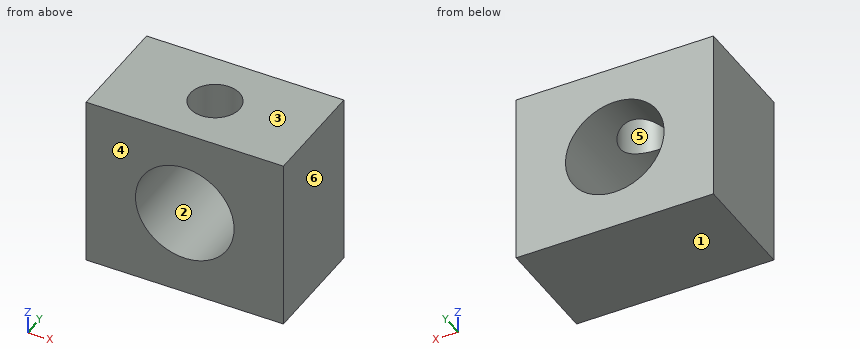
```python
from build123d import *

# Parameters (mm, degrees)
F0_W     = 80
F0_H     = 70
F1_DEPTH = 45
F2_R     = 20
F3_DEPTH = 45.001
F4_R     = 10
F5_DEPTH = 25


with BuildPart() as f1:
    # F0 (on Front) → F1 (new body)
    with BuildSketch(Plane.XZ):
        Rectangle(F0_W, F0_H)
    extrude(amount=-F1_DEPTH)

    # F2 (on face) → F3 (cut, through all)
    with BuildSketch(Plane.XZ):
        Circle(F2_R)
    extrude(amount=-F3_DEPTH, mode=Mode.SUBTRACT)

    # F4 (on face) → F5 (cut)
    with BuildSketch(Plane.XY.offset(35)):
        with Locations((0, 22.5)):
            Circle(F4_R)
    extrude(amount=-F5_DEPTH, mode=Mode.SUBTRACT)


solid = f1.part
```
Geometry: final body of the model. Coordinates: model frame, mm. Face numbers are marked on the shaded views. A direction names the side the tool comes from. Coordinates: 2 decimals unless noted, no trailing zeros. Write each loop counter-clockwise with the first axis right and the second up, starting at its lowest first coordinate (ties: lowest second). Pieces come first, ordered by that corner, then holes. Notation, with made-up numbers: M 14.25,-33 L 41.25,-33 A16 cw 41.25,-29 Z; hole C 56.25,-24.5 d6. An arc over 180 degrees is marked long. Use CSV: the item, a comma, the result in double quotes. Start each with the question number.
1. Cut plane C-C on y = 22.5. Return the cut outline in (x, z).
2. Mould query, pull axis Z, two halves, no side actions, for the marked faces 1, 2, 3 and 4. Classes: pulls with the +Z half, pulls with the -Z half, needs draft (parallel to the pull), parting line crosses it, or undercut.
3. Reachability of the marked faces 5 and 6 from +Z, -Z, +X, -X, +Y, -Y: full face, straight path, thin tool, end or side. Return the list, or none.
4. Cut plane D-D on x = -17.5. Return the cut outline in (y, z), plus the area to 3 significant figures.
5. Cut plane B-B on x = 0. Return the cut outline in (y, z), plus the area to 3 significant figures.
6. Cut plane A-A on z = 0. Return the cut outline in (x, y).
7. Ray query, probe 1 along Z at (x, y) = (0, 36); probe 2 along X at (y, z) = (22.5, 27.5); probe 3 along Y at (x, z) = (0, 25). Return the intervals inside material, ascending.
Entries:
1,outline,"M -40,-35 L 40,-35 L 40,35 L 10,35 L 10,17.32 A20 cw long -10,17.32 L -10,35 L -40,35 Z"
2,face 1,"pulls with the -Z half"
2,face 2,"undercut"
2,face 3,"pulls with the +Z half"
2,face 4,"needs draft"
3,face 5,"+Z"
3,face 6,"+Z, -Z, +X, +Y, -Y"
4,outline,"M 0,-35 L 45,-35 L 45,-9.68 L 0,-9.68 Z; M 0,9.68 L 45,9.68 L 45,35 L 0,35 Z"
4,area,"2,280 mm²"
5,outline,"M 0,-35 L 45,-35 L 45,-20 L 0,-20 Z; M 0,20 L 12.5,20 L 12.5,35 L 0,35 Z; M 32.5,20 L 45,20 L 45,35 L 32.5,35 Z"
5,area,"1,050 mm²"
6,outline,"M -40,0 L -20,0 L -20,45 L -40,45 Z; M 20,0 L 40,0 L 40,45 L 20,45 Z"
7,probe 1,"-35 to -20, 20 to 35"
7,probe 2,"-40 to -10, 10 to 40"
7,probe 3,"0 to 12.5, 32.5 to 45"
